The model under review builds one solid part; all positions refer to its coordinate system, in mm. Face numbers are marked on the shaded views. A direction names the side the tool comes from. Coordinates: 2 decimals unless noted, no trailing zeros. Order: outer loops, then holes, each group sorted by start corner. A loop starts at its lowest first (then second) coordinate and runs counter-clockwise, first axis right, second up. Notation, with made-up numbers: M 26.5,-30.5 L 59.5,-30.5 A25 ccw 59.5,6.5 Z; hole C 23.25,81.5 d1. An arc over 180 degrees is marked long. Answer in a Markdown table with one row per item.
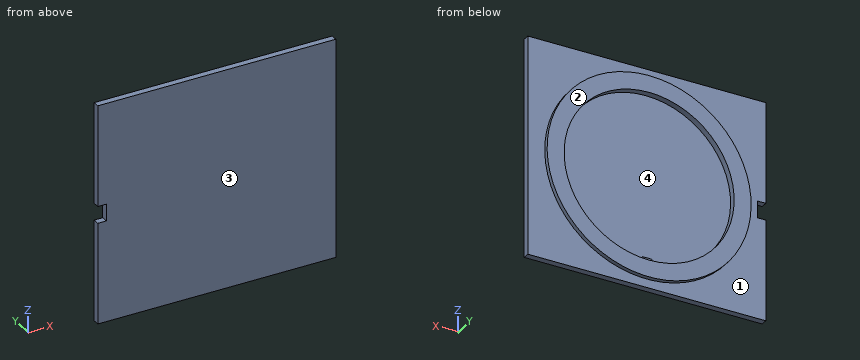
from build123d import *

# Parameters (mm, degrees)
SKETCH1_R           = 24
SKETCH1_R_2         = 20
BOSS_EXTRUDE1_DEPTH = 2.5
SKETCH2_R           = 24
BOSS_EXTRUDE2_DEPTH = 1
SKETCH3_W           = 56
SKETCH3_H           = 52
SKETCH3_R           = 24
BOSS_EXTRUDE3_DEPTH = 1.5
BOSS_EXTRUDE4_DEPTH = 0.6
CHAMFER1_SIZE       = 0.5
SKETCH5_W           = 18.188296091
SKETCH5_H           = 4
CUT_EXTRUDE1_DEPTH  = 39.291643997


with BuildPart() as part:
    # Sketch1 → Boss-Extrude1 (new body)
    with BuildSketch(Plane(origin=(0, 0, 0), x_dir=(1, 0, 0), z_dir=(0, 1, 0))):
        with Locations(Location((0, 0, 0), (0, 0, 270))):
            Circle(SKETCH1_R)
        with Locations(Location((0, 0, 0), (0, 0, 270))):
            Circle(SKETCH1_R_2, mode=Mode.SUBTRACT)
    extrude(amount=BOSS_EXTRUDE1_DEPTH)

    # Sketch2 → Boss-Extrude2 (add)
    with BuildSketch(Plane.XZ):
        with Locations(Location((0, 0, 0), (0, 0, 90))):
            Circle(SKETCH2_R)
    extrude(amount=-BOSS_EXTRUDE2_DEPTH)

    # Sketch3 → Boss-Extrude3 (add)
    with BuildSketch(Plane.XZ):
        Rectangle(SKETCH3_W, SKETCH3_H)
        with Locations(Location((0, 0, 0), (0, 0, 270))):
            Circle(SKETCH3_R, mode=Mode.SUBTRACT)
    extrude(amount=-BOSS_EXTRUDE3_DEPTH)

    # Sketch4 → Boss-Extrude4 (add)
    with BuildSketch(Plane(origin=(0, 1, 0), x_dir=(1, 0, 0), z_dir=(0, 1, 0))):
        with BuildLine():
            Line((1.5, 19), (1.5, 19.943670675))
            ThreePointArc((1.5, 19.943670675), (0, 20), (-1.5, 19.943670675))
            Line((-1.5, 19.943670675), (-1.5, 19))
            Line((-1.5, 19), (1.5, 19))
        make_face()
    extrude(amount=BOSS_EXTRUDE4_DEPTH)

    # Chamfer1
    chamfer1_edges = [part.edges().sort_by_distance(p)[0] for p in [
        (-1.5, 1.3, -19),
        (1.5, 1.3, -19),
    ]]
    chamfer(chamfer1_edges, length=CHAMFER1_SIZE)

    # Sketch5 → Cut-Extrude1 (cut, through all)
    with BuildSketch(Plane.XZ):
        with Locations((-35.094148046, 0)):
            Rectangle(SKETCH5_W, SKETCH5_H)
    extrude(amount=-CUT_EXTRUDE1_DEPTH, mode=Mode.SUBTRACT)


solid = part.part
(1) Take a section at C-C (x = -11). Write out the cut boundary in (y, z).
Report:
| item | result |
|---|---|
| outline | M 0,-26 L 1.5,-26 L 1.5,-21.33 L 2.5,-21.33 L 2.5,-16.7 L 1,-16.7 L 1,16.7 L 2.5,16.7 L 2.5,21.33 L 1.5,21.33 L 1.5,26 L 0,26 Z |
(2) Take a section at D-D (z = 22). Write out the cut boundary in (x, y), then the cut area to 3 significant figures.
Report:
| item | result |
|---|---|
| outline | M -28,0 L 28,0 L 28,1.5 L 9.59,1.5 L 9.59,2.5 L -9.59,2.5 L -9.59,1.5 L -28,1.5 Z |
| area | 103 mm^2 |
(3) To check wall thickness, follow line 1 (Z direction, x = 0, y = 2.25); line 2 (Z direction, x = 0, y = 1.3). State the ranges of each line that lie inside material, in increasing order. Write a range as [from, to].
Report:
| item | result |
|---|---|
| line 1 | [-24, -20], [20, 24] |
| line 2 | [-26, -19], [20, 26] |
(4) Insertion check: P1, Ø12, axis at x = -5.5, z = -7.5, coming from the +Y side; P2, Ø1.2, axis at y = 0.5, z = 0.5, coming from the -X side; P3, Ø0.8, axis at x = 0.5, z = -19.5, coming from the +Y side. Each pin has a flat end and moves straight along its axis. Give the tip position at first contact, or say it passes through.
Report:
| item | result |
|---|---|
| P1 | y = 1 |
| P2 | x = -26 |
| P3 | y = 1.6 |
(5) The part is to be moulded in two halves that separate along Z. For the marked faces 3 and 4, say which applies: +Z half, -Z half, draft (parallel to the pull), parting line (faces both ways), or undercut.
Report:
| item | result |
|---|---|
| face 3 | draft |
| face 4 | undercut |
(6) Take a section at A-A (z = 0). Write out the cut boundary in (x, y), then the cut area to 3 significant figures.
Report:
| item | result |
|---|---|
| outline | M -26,0 L 28,0 L 28,1.5 L 24,1.5 L 24,2.5 L 20,2.5 L 20,1 L -20,1 L -20,2.5 L -24,2.5 L -24,1.5 L -26,1.5 Z |
| area | 69.0 mm^2 |
(7) Take a section at B-B (x = 0). Write out the cut boundary in (y, z), then the cut area to 3 significant figures.
Report:
| item | result |
|---|---|
| outline | M 0,-26 L 1.5,-26 L 1.5,-24 L 2.5,-24 L 2.5,-20 L 1.6,-20 L 1.6,-19 L 1,-19 L 1,20 L 2.5,20 L 2.5,24 L 1.5,24 L 1.5,26 L 0,26 Z |
| area | 66.6 mm^2 |
(8) Machinability: for the marked faces 1 and 2, which of the approach directions +Z, -Z, +X, -X, +Y, -Y give a long, thin tool a straight path to every point of the face, cutting with its end or side? Answer none if there is none.
Report:
| item | result |
|---|---|
| face 1 | +Y |
| face 2 | +Z, -Z, +X, -X, +Y |
